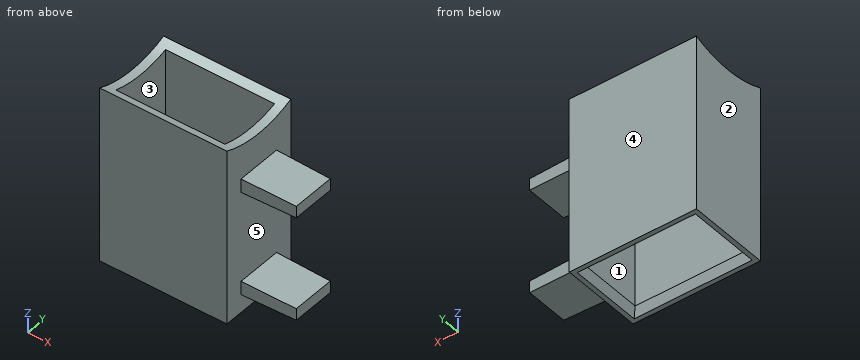
```python
from build123d import *

# Parameters (mm, degrees)
SKETCH9_W                     = 12
SKETCH9_H                     = 7
BOSS_EXTRUDE5_DEPTH           = 25
SHELL6_T                      = 1
CUT_EXTRUDE2_REACH            = 31.004
SKETCH12_R                    = 11.5
SKETCH14_W                    = 14
SKETCH14_H                    = 9
SKETCH14_W_2                  = 12
SKETCH14_H_2                  = 7
BOSS_EXTRUDE6_DEPTH           = 5
CHAMFER2_SIZE                 = 0.5
CHAMFER2_SIZE2                = 0.866025404
SKETCH16_W                    = 5
SKETCH16_H                    = 1.5
BOSS_EXTRUDE7_DEPTH           = 6
BOSS_EXTRUDE7_DRAFT           = 1
BOSS_EXTRUDE7_PROFILE_2_DEPTH = 6
BOSS_EXTRUDE7_PROFILE_2_DRAFT = 1
BODY_MOVE_COPY1_ANGLE         = 90


with BuildPart() as part:
    # Sketch9 → Boss-Extrude5 (new body)
    with BuildSketch(Plane(origin=(0, 0, 0), x_dir=(1, 0, 0), z_dir=(0, 1, 0))):
        Rectangle(SKETCH9_W, SKETCH9_H)
    extrude(amount=BOSS_EXTRUDE5_DEPTH)

    # Shell6
    shell6_openings = [part.faces().sort_by_distance(p)[0] for p in [
        (0, 0, 0),
        (0, 25, 0),
    ]]
    offset(amount=SHELL6_T, openings=shell6_openings, kind=Kind.INTERSECTION)

    # Sketch12 → Cut-Extrude2 (cut, up to next)
    with BuildSketch(Plane(origin=(7, 0, 0), x_dir=(0, 0, -1), z_dir=(1, 0, 0)), mode=Mode.PRIVATE) as cut_extrude2_sk1:
        Circle(SKETCH12_R)
    cut_extrude2_tool1 = extrude(cut_extrude2_sk1.sketch, amount=-CUT_EXTRUDE2_REACH, mode=Mode.PRIVATE) & part.part
    add(cut_extrude2_tool1.solids().sort_by_distance((7, 0, 0))[0], mode=Mode.SUBTRACT)

    # Sketch14 → Boss-Extrude6 (add)
    with BuildSketch(Plane(origin=(0, 25, 0), x_dir=(1, 0, 0), z_dir=(0, 1, 0))):
        Rectangle(SKETCH14_W, SKETCH14_H)
        Rectangle(SKETCH14_W_2, SKETCH14_H_2, mode=Mode.SUBTRACT)
    extrude(amount=BOSS_EXTRUDE6_DEPTH)

    # Chamfer2
    chamfer2_edges = [part.edges().sort_by_distance(p)[0] for p in [
        (6, 30, 0),
        (0, 30, -3.5),
        (-6, 30, 0),
        (0, 30, 3.5),
    ]]
    chamfer2_side = [part.faces().sort_by_distance(p)[0] for p in [
        (0, 30, -4.33356683),
    ]]
    chamfer(chamfer2_edges, length=CHAMFER2_SIZE, length2=CHAMFER2_SIZE2, reference=chamfer2_side[0])


with BuildPart() as boss_extrude7_tool:
    # Sketch16 → Boss-Extrude7 (with draft: the straight prism first)
    with BuildSketch(Plane(origin=(7, 0, 0), x_dir=(0, 0, -1), z_dir=(1, 0, 0))):
        with Locations((0, 27.25)):
            Rectangle(SKETCH16_W, SKETCH16_H)
    extrude(amount=BOSS_EXTRUDE7_DEPTH)
    # Boss-Extrude7: the draft: its side faces are tilted about the plane it starts from
    boss_extrude7_sides = [boss_extrude7_tool.faces().sort_by_distance(p)[0] for p in [
        (10, 27.25, 2.5),
        (10, 26.5, 0),
        (10, 27.25, -2.5),
        (10, 28, 0),
    ]]
    draft(boss_extrude7_sides, Plane(origin=(7, 0, 0), x_dir=(0, 0, -1), z_dir=(1, 0, 0)), BOSS_EXTRUDE7_DRAFT)


with BuildPart() as part_1:
    add(part.part)

    # Boss-Extrude7: add boss_extrude7_tool
    add(boss_extrude7_tool.part)


with BuildPart() as boss_extrude7_profile_2_tool:
    # Sketch16 → Boss-Extrude7 profile 2 (with draft: the straight prism first)
    with BuildSketch(Plane(origin=(7, 0, 0), x_dir=(0, 0, -1), z_dir=(1, 0, 0))):
        with Locations((0, 15.75)):
            Rectangle(SKETCH16_W, SKETCH16_H)
    extrude(amount=BOSS_EXTRUDE7_PROFILE_2_DEPTH)
    # Boss-Extrude7 profile 2: the draft: its side faces are tilted about the plane it starts from
    boss_extrude7_profile_2_sides = [boss_extrude7_profile_2_tool.faces().sort_by_distance(p)[0] for p in [
        (10, 15.75, 2.5),
        (10, 15, 0),
        (10, 15.75, -2.5),
        (10, 16.5, 0),
    ]]
    draft(boss_extrude7_profile_2_sides, Plane(origin=(7, 0, 0), x_dir=(0, 0, -1), z_dir=(1, 0, 0)), BOSS_EXTRUDE7_PROFILE_2_DRAFT)


with BuildPart() as part_2:
    add(part_1.part)

    # Boss-Extrude7 profile 2: add boss_extrude7_profile_2_tool
    add(boss_extrude7_profile_2_tool.part)


with BuildPart() as part_3:
    # Body-Move/Copy1: moved
    add(part_2.part.rotate(Axis((0, 20.291502622, 0), (-1, 0, 0)), BODY_MOVE_COPY1_ANGLE))


solid = part_3.part
```
Model file for the job. Use its own axes, mm. Face numbers are marked on the shaded views. A direction names the side the tool comes from. Coordinates: 2 decimals unless noted, no trailing zeros. Order: outer loops, then holes, each group sorted by start corner. A loop starts at its lowest first (then second) coordinate and runs counter-clockwise, first axis right, second up. Notation, with made-up numbers: (60.5, -12.75) - (83.5, -12.75) arc R24 cw to (83.5, 1.25) - close; hole circle Ø1 at (27.25, 64). An arc over 180 degrees is marked (long way). Return JSON: item names as keys, results as strings. Group by question number.
1) Probe line 1 (Y direction, x = 0.75, z = 8.5); line 2 (X direction, y = 17.75, z = -6); line 3 (X direction, y = 20.5, z = 4.5). List the from-to ranges inside material, lowest first. Write a range as from..to.
2) Mould opens along X. For the marked faces 3, 4 and 5 say: released by +X, released by -X, zero draft, split by the parting line, or undercut.
3) Saw through at A-A, the plane z = -0.75. Write the cut outline in (x, y).
4) Flat gauge pin, fed straight in: P1, Ø4, axis at x = 4, y = 22, coming from the -Z side. Where does the tip first touch, or does it go through?
5) Saw through at C-C, the plane y = 23.25. Write the cut outline in (x, z), plus the area to 3 significant figures.
6) Saw through at B-B, the plane x = 4. Write the cut outline in (y, z).
7) Tool access for the marked faces 1 and 2: list every direction of +Z, -Z, +X, -X, +Y, -Y with a clear straight run to the whole face (end or side of a thin tool).
8) Saw through at D-D, the plane y = 21.75. Write the cut outline in (x, z).
Values found:
{
 "1": {"line 1": "y = 15.79..16.79, 23.79..24.79", "line 2": "x = -7..-6, 6..7", "line 3": "x = -7..-6, 6..13"},
 "2": {"face 3": "undercut", "face 4": "zero draft", "face 5": "released by +X"},
 "3": {"outline": "(-7, 15.79) - (7, 15.79) - (7, 24.79) - (-7, 24.79) - close; hole (-6, 16.79) - (6, 16.79) - (6, 23.79) - (-6, 23.79) - close"},
 "4": {"P1": "stops at z = -9.2"},
 "5": {"outline": "(-7, -9.71) - (-6.5, -9.71) - (-6, -8.84) - (-6, 9.18) - (-7, 9.18) - close; (6, -8.84) - (6.5, -9.71) - (7, -9.71) - (7, 9.18) - (6, 9.18) - close", "area": "37.3 mm²"},
 "6": {"outline": "(15.79, -9.71) - (16.29, -9.71) - (16.79, -8.84) - (16.79, 9.34) arc R11.5 cw to (15.79, 9.71) - close; (23.79, -8.84) - (24.29, -9.71) - (24.79, -9.71) - (24.79, 9.71) arc R11.5 cw to (23.79, 9.34) - close"},
 "7": {"face 1": "+Z, -Z", "face 2": "+Z, -Z, -X, +Y, -Y"},
 "8": {"outline": "(-7, -9.71) - (-6.5, -9.71) - (-6, -8.84) - (-6, 8.88) - (-7, 8.88) - close; (6, -8.84) - (6.5, -9.71) - (7, -9.71) - (7, -7.71) - (13, -7.6) - (13, -6.31) - (7, -6.21) - (7, 3.79) - (13, 3.9) - (13, 5.19) - (7, 5.29) - (7, 8.88) - (6, 8.88) - close"}
}
